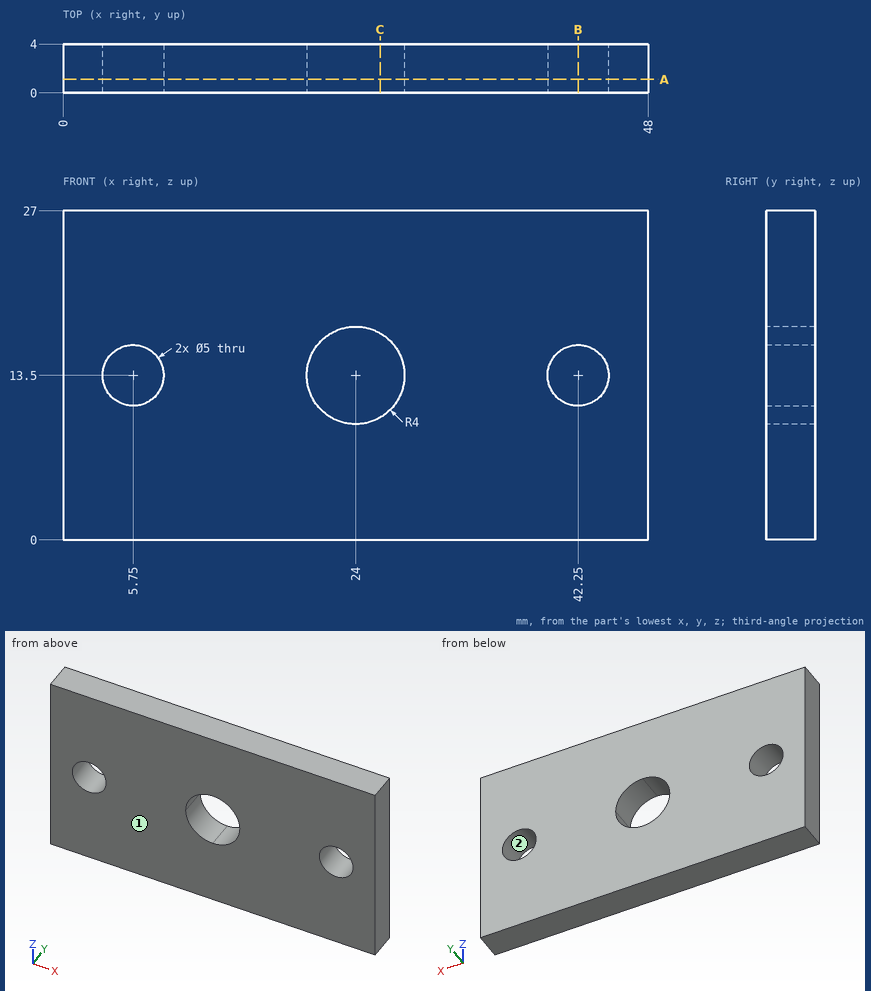
Source: three-view drawing plus pictorial views. Frame: mm from the lowest corner of the part. Round coordinates to 2 decimals unless told otherwise and drop trailing zeros. Order: outer loops, then holes, each group sorted by start corner. A loop starts at its lowest first (then second) coordinate and runs counter-clockwise, first axis right, second up. Notation, with made-up numbers: (61, -11) - (101, -11) arc R20 ccw to (101, -4) - close; hole circle Ø5 at (83, 9). An arc over 180 degrees is marked (long way). Answer in a Markdown table with one row per item.
Item 1: Section query A-A (y = 1.1). Return the cut outline in (x, z).
Model answer:
| item | result |
|---|---|
| outline | (0, 0) - (48, 0) - (48, 27) - (0, 27) - close; hole circle Ø5 at (5.75, 13.5); hole circle Ø8 at (24, 13.5); hole circle Ø5 at (42.25, 13.5) |
Item 2: Mould query, pull axis X, two halves, no side actions, for the marked faces 1 and 2. Classes: released by +X, released by -X, zero draft, split by the parting line, or undercut.
Model answer:
| item | result |
|---|---|
| face 1 | zero draft |
| face 2 | undercut |
Item 3: Section query C-C (x = 26). Return the cut outline in (y, z), then the cut area to 3 significant figures.
Model answer:
| item | result |
|---|---|
| outline | (0, 0) - (4, 0) - (4, 10.04) - (0, 10.04) - close; (0, 16.96) - (4, 16.96) - (4, 27) - (0, 27) - close |
| area | 80.3 mm² |
Item 4: Line query: line 1 (Z direction, x = 5.75, y = 1.5); line 2 (X direction, y = 3.4, z = 15.5); line 3 (X direction, y = 0.65, z = 12.5). Output: solid intervals per line, ascending.
Model answer:
| item | result |
|---|---|
| line 1 | z = 0 to 11, 16 to 27 |
| line 2 | x = 0 to 4.25, 7.25 to 20.54, 27.46 to 40.75, 43.75 to 48 |
| line 3 | x = 0 to 3.46, 8.04 to 20.13, 27.87 to 39.96, 44.54 to 48 |
Item 5: Section query B-B (x = 42.25). Return the cut outline in (y, z).
Model answer:
| item | result |
|---|---|
| outline | (0, 0) - (4, 0) - (4, 11) - (0, 11) - close; (0, 16) - (4, 16) - (4, 27) - (0, 27) - close |
